Model file for the job. Use its own axes, mm. Face numbers are marked on the shaded views. Round coordinates to 2 decimals unless told otherwise and drop trailing zeros. Order: outer loops, then holes, each group sorted by start corner. A loop starts at its lowest first (then second) coordinate and runs counter-clockwise, first axis right, second up. Notation, with made-up numbers: (75, -37) -> (101, -37) arc R16 cw to (101, -12) -> close; hole circle Ø3 at (-9.5, -6.75). An arc over 180 degrees is marked (long way). Put each result on its own line as item: value. Start each with the question number.
Q1. Cut at A-A, the plane x = 34. List the corners of the cut face in (y, z).
Q2. Pull direction Y, two halves, no side cores. Call the marked faces 1, 2 and 3: released by +Y, released by -Y, zero draft, split by the parting line, or undercut.
Q3. Probe L1, parallel to Z at x = 42, y = 0; L2, parallel to X at y = 2.5, z = 3.75; L3, parallel to Z at x = 6, y = -3.5. List the from-to ranges inside material, lowest first.
Q4. Flat gauge pins, fed straight in: P1, Ø3, axis at y = 1, z = 4.5, coming from the +X side; P2, Ø1.4, axis at x = -3, z = 0.5, coming from the -Y side; P3, Ø4, axis at x = 38, y = -5.5, coming from the +Z side; P4, Ø1.5, axis at x = 40, z = -1.5, coming from the +Y side. Where does each tip first touch, or does it go through?
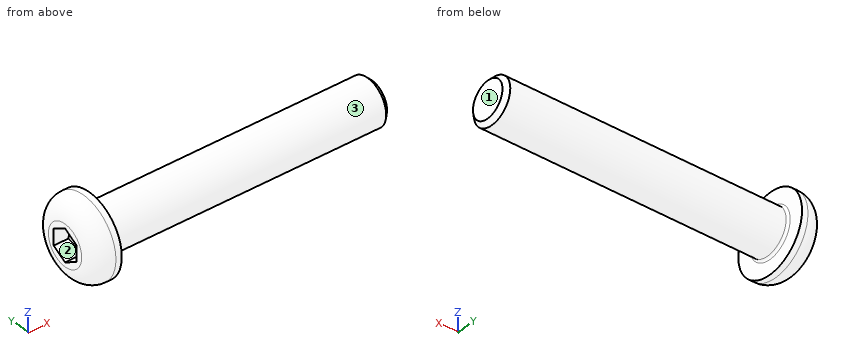
Autodesk Inventor part; units mm, degrees
ref_plane "Work Plane1" through (29, 0, 0) normal (0, -1, 0) x (1, 0, 0)
ref_plane "YZ Plane" through (0, 0, 0) normal (1, 0, 0) x (0, 1, 0)
ref_plane "XZ Plane" through (0, 0, 0) normal (0, 1, 0) x (-1, 0, 0)
sketch "Sketch1" plane through (0, 0, 0) normal (0, 0, 1) x (1, 0, 0)
  line L0 (-0.1333, 0) -> (50, 0)
  line L1 (50, 0) -> (50, 4)
  line L2 (50, 4) -> (22, 4)
  line L3 (22, 4) -> (21.2331, 4)
  line L4 (21.2331, 4) -> (0, 4)
  line L5 (0, 4) -> (0, 7)
  line L6 (0, 7) -> (-4.4, 7)
  line L7 (-4.4, 7) -> (-4.4, 2.8868)
  line L8 (-4.4, 2.8868) -> (-1.8, 2.8868)
  line L9 (-1.8, 2.8868) -> (-0.1333, 0)
  line L10 (-15.28, 0) -> (60.88, 0)
  line L11 (0, -1.4) -> (0, 8.4)
  line L12 (22, 4) -> (0, 4) construction
  dimension "d1" = 28
  dimension "d2" = 0.7669
  dimension "d3" = 4.4
  dimension "d4" = 2.6
  dimension "d5" = 60
  dimension "d6" = 8
  dimension "d7" = 8
  dimension "d8" = 5.7735
  dimension "d9" = 14
  dimension "d26" = 50
revolve "Body" add sketch "Sketch1" angle 360 about axis through (-0.1333, 0, 0) along (1, 0, 0)
sketch "Sketch2" plane through (-4.4, 0, 0) normal (-1, 0, 0) x (0, 0, 1)
  circle A0 centre (0, 0) radius 2.8868
  line L0 (0, -9.8) -> (0, 9.8)
  line L1 (-9.8, 0) -> (9.8, 0)
  line L2 (2.8868, 0) -> (1.4434, -2.5)
  line L3 (1.4434, -2.5) -> (-1.4434, -2.5)
  line L4 (-1.4434, -2.5) -> (-2.8868, 0)
  line L5 (-2.8868, 0) -> (-1.4434, 2.5)
  line L6 (-1.4434, 2.5) -> (1.4434, 2.5)
  line L7 (1.4434, 2.5) -> (2.8868, 0)
extrude "Slot" add sketch "Sketch2" against normal up to next contours L7 A0 | A0 L2 | L6 L0 A0 | A0 L0 L3 | L0 L6 A0 | A0 L3 L0 | L4 A0 | A0 L5
fillet "Fillet1" radius 3.35 1 edges at (-4.4, -7, 0)
thread "Thread"
chamfer "Chamfer1" distance 0.7668 distance2 0.7668 1 edges at (50, -4, 0) measured on face at (50, -0.3588, -0.308)
ref_plane "Work Plane1" through (29, 0, 0) normal (0, -1, 0) x (1, 0, 0)
fillet "Fillet2" radius 0.4 1 edges at (0, -4, 0)
equation "\"d1\" = GEL"
equation "\"d3\" = KOH"
equation "\"d4\" = INTI"
equation "\"d6\" = GD"
equation "\"d7\" = BDM"
equation "\"d8\" = 1.1547 * SW"
equation "\"d9\" = KOD"
equation "\"d26\" = NLG"
equation "\"d30\" = R"
equation "\"d17\" = RR"
equation "\"d13\" = GEL"
equation "\"d15\" = -0.5 * SPD + 0.5 * GD"
equation "\"d16\" = GUL"
equation "\"GD\" = NND"
equation "\"NLG\" = 50"
equation "\"GEL\" = 28"
equation "\"KOD\" = 14"
equation "\"KOH\" = 4.4"
equation "\"INTI\" = 2.6"
equation "\"GAL\" = 0.61345 * PTC"
equation "\"GUL\" = 0.61345 * PTC"
equation "\"BDM\" = NND"
equation "\"SW\" = 5"
equation "\"RR\" = 3.35"
equation "\"SPD\" = NND - 1.2269 * PTC"
equation "\"R\" = 0.4"
equation "\"TOA\" = 30deg"
equation "\"GD1\" = THREADDIA - 1.2269 * PTC"
equation "\"THREADDIA\" = 8"
equation "\"PTC\" = 1.25"
equation "\"NND\" = 8"
equation "\"KOH1\" = 1.05"
equation "\"E0\" = 5.723"
properties part number "PWTR-0132" material "Stainless Steel"
Ans:
1. outline: circle Ø8 at (0, 0)
2. face 1: zero draft
2. face 2: undercut
2. face 3: split by the parting line
3. L1: z = -4 to 4
3. L2: x = -4.29 to 0
3. L3: z = -1.94 to 1.94
4. P1: stops at x = 50
4. P2: stops at y = -6.74
4. P3: stops at z = 1.94
4. P4: stops at y = 3.93
